The model under review builds one solid part; all positions refer to its coordinate system, in mm. A direction names the side the tool comes from. Coordinates: 2 decimals unless noted, no trailing zeros. Write each loop counter-clockwise with the first axis right and the second up, starting at its lowest first coordinate (ties: lowest second). Pieces come first, ordered by that corner, then holes. Notation, with made-up numbers: M 73.5,7 L 114.5,7 A24 ccw 114.5,39 Z; hole C 36,-7 d5. An arc over 180 degrees is marked long. Answer as a JSON object with one key per item and string values.
```python
from build123d import *

# Parameters (mm, degrees)
F1_DEPTH  = 16
F2_W      = 70
F2_H      = 3
F3_DEPTH  = 2
F4_W      = 50
F4_H      = 14
F5_DEPTH  = 2
F6_R      = 1
F9_DEPTH  = 2
F11_DEPTH = 42.001


with BuildPart() as f1:
    # F0 (on Front) → F1 (new body)
    with BuildSketch(Plane.XZ):
        with BuildLine():
            Line((94, 9), (0, 9))
            ThreePointArc((0, 9), (-9, 0), (0, -9))
            Line((0, -9), (15.2698143006, -9))
            ThreePointArc((15.2698143006, -9), (18.2087071496, -9.9548907528), (20.0250713566, -12.4548364712))
            ThreePointArc((20.0250713566, -12.4548364712), (41.226339877, -44.1268775333), (75.8783002618, -59.9967739854))
            ThreePointArc((75.8783002618, -59.9967739854), (80.6596281551, -61.5636317865), (84.7179401809, -64.5378952739))
            Line((84.7179401809, -64.5378952739), (86.0083877193, -62.9999997839))
            ThreePointArc((86.0083877193, -62.9999997839), (81.4277187811, -59.7105770288), (76.0540091245, -57.9999997839))
            ThreePointArc((76.0540091245, -57.9999997839), (42.4723911749, -42.5610388699), (21.9271739736, -11.8367711264))
            ThreePointArc((21.9271739736, -11.8367711264), (19.3842641622, -8.3368472287), (15.2698143006, -7.0000002161))
            Line((15.2698143006, -7.0000002161), (0, -7.0000002161))
            ThreePointArc((0, -7.0000002161), (-7.0000002161, 0), (0, 7.0000002161))
            Line((0, 7.0000002161), (94, 7.0000002161))
            Line((94, 7.0000002161), (94, 9))
        make_face()
    extrude(amount=F1_DEPTH)

    # F2 (on face) → F3 (join)
    with BuildSketch(Plane.XY.offset(9)):
        with Locations((59, -17.5)):
            Rectangle(F2_W, F2_H)
    extrude(amount=-F3_DEPTH)

    # F4 (on face) → F5 (join)
    with BuildSketch(Plane.XZ.offset(19)):
        with Locations((69, 2)):
            Rectangle(F4_W, F4_H)
    extrude(amount=F5_DEPTH)

    # F6
    f6_edges = [f1.edges().sort_by_distance(p)[0] for p in [
        (69, -21, 9),
        (69, -19, 7),
    ]]
    fillet(f6_edges, radius=F6_R)

    # F7: F1 across plane


with BuildPart() as f1_1:
    add(f1.part)
    add(f1.part.mirror(Plane.XZ))

    # F8 (on face) → F9 (cut)
    with BuildSketch(Plane.XY.offset(9)):
        with BuildLine():
            Line((94, 12), (34, 12))
            ThreePointArc((34, 12), (22, 0), (34, -12))
            Line((34, -12), (94, -12))
            Line((94, -12), (94, 12))
        make_face()
    extrude(amount=-F9_DEPTH, mode=Mode.SUBTRACT)

    # F10 (on face) → F11 (cut, through all)
    with BuildSketch(Plane.XZ.offset(21)):
        with BuildLine():
            ThreePointArc((50, 3), (47, 0), (50, -3))
            Line((50, -3), (70, -3))
            ThreePointArc((70, -3), (73, 0), (70, 3))
            Line((70, 3), (50, 3))
        make_face()
    extrude(amount=-F11_DEPTH, mode=Mode.SUBTRACT)


solid = f1_1.part
```
(1) For pin 1 Ø22 at (x, z) = (25.5, -43.5) entering from +Y; pin 2 Ø1.5 at (x, y) = (47.5, -18) entering from -Z; pin 3 Ø2 at (x, z) = (29.5, 8) entering from +Y, all flat-tipped, find the tip position at first contact; note any pin that passes through.
Results list:
{"pin 1": "y = 16", "pin 2": "z = 6.66", "pin 3": "y = 19"}
(2) Wall thickness on line 1 along Z through (x, y) = (11, 1.5); line 2 along Y through (x, z) = (39, -40.5); line 3 along Z through (x, y) = (18, 11): over which ranges is each line inside the solid? List them lowest first. Write a range as from..to.
Results list:
{"line 1": "-9..-7, 7..9", "line 2": "-16..16", "line 3": "-9.81..-7.55, 7..9"}
(3) Add section D-D on x = 81. Give the boundary of the cut face in (y, z), and give its area (3 significant figures).
Results list:
{"outline": "M -21,-5 L -19,-5 L -19,6 A1 cw -18,7 L -12,7 L -12,9 L -20,9 A1 ccw -21,8 Z; M -16,-61.74 L 16,-61.74 L 16,-59.5 L -16,-59.5 Z; M 12,7 L 18,7 A1 cw 19,6 L 19,-5 L 21,-5 L 21,8 A1 ccw 20,9 L 12,9 Z", "area": "156 mm²"}
(4) Add section B-B on y = 0. Give the boundary of the cut face in (x, z).
Results list:
{"outline": "M 0,-9 L 15.27,-9 A5 cw 20.03,-12.45 A70 ccw 75.88,-60 A16 cw 84.72,-64.54 L 86.01,-63 A18 ccw 76.05,-58 A68 cw 21.93,-11.84 A7 ccw 15.27,-7 L 0,-7 A7 cw 0,7 L 22,7 L 22,9 L 0,9 A9 ccw Z"}
(5) Draft analysis for pull direction Z (two halves, no side actions). For faces 1 (the face through (8, 0, -7)), 2 (the face through (94, 19.5, 4.6)), 3 (the face through (18.173, -0.224, -9.929)), state which applies: released by +Z, released by -Z, zero draft, split by the parting line, or undercut.
Results list:
{"face 1": "undercut", "face 2": "zero draft", "face 3": "released by -Z"}
(6) Add section C-C on x = 67. Give the boundary of the cut face in (y, z), and give its area (3 significant figures).
Results list:
{"outline": "M -21,-5 L -19,-5 L -19,-3 L -21,-3 Z; M -21,3 L -19,3 L -19,6 A1 cw -18,7 L -12,7 L -12,9 L -20,9 A1 ccw -21,8 Z; M -16,-58.02 L 16,-58.02 L 16,-55.94 L -16,-55.94 Z; M 12,7 L 18,7 A1 cw 19,6 L 19,3 L 21,3 L 21,8 A1 ccw 20,9 L 12,9 Z; M 19,-5 L 21,-5 L 21,-3 L 19,-3 Z", "area": "127 mm²"}
(7) For faces 4 (the face through (74, 19, 1)), 5 (the face through (22, 0, 8)), 6 (the face through (42.87, -0.22, -42.9)), list the 3-axis set-ups (+Z, -Z, +X, -X, +Y, -Y) from which the entire face can be reached by the end or side of a thin tool; tool diameter is ignored.
Results list:
{"face 4": "-Z, +X, -X", "face 5": "+Z, +X", "face 6": "+X, +Y, -Y"}
(8) Add section A-A on z = 0. Give the boundary of the cut face in (x, y).
Results list:
{"outline": "M -9,-16 L -7,-16 L -7,16 L -9,16 Z; M 44,-21 L 47,-21 L 47,-19 L 44,-19 Z; M 44,19 L 47,19 L 47,21 L 44,21 Z; M 73,-21 L 94,-21 L 94,-19 L 73,-19 Z; M 73,19 L 94,19 L 94,21 L 73,21 Z"}
